from build123d import *

# Parameters (mm, degrees)
F1_DEPTH    = 6
F2_F1_R     = 0.2
F2_F2_R     = 0.2
F3_T4_DEPTH = 28.4585903453
F3_T9_DEPTH = 28.4585903453
F4_R        = 5.99999


# Not quite as in the source:
# - a fillet or chamfer that OpenCascade refuses, or shapes differently, is made with other operations: its cross-section is extruded or revolved along the edge and cut away or added
# - a fillet or chamfer is up to 0.001 mm smaller than in the source, because OpenCascade refuses the exact size


with BuildPart() as f1:
    # F0 (on Top) → F1 (new body)
    with BuildSketch(Plane.XY):
        Polygon((-7.5, 8), (-4.418584287, -3.5), (4.418584287, -3.5), (7.5, 8), align=None)
        with BuildLine():
            ThreePointArc((-1.5, 1.5), (-2.5606601718, 4.0606601718), (0, 3))
            ThreePointArc((0, 3), (2.5606601718, 4.0606601718), (1.5, 1.5))
            ThreePointArc((1.5, 1.5), (2.5606601718, -1.0606601718), (0, 0))
            ThreePointArc((0, 0), (-2.5606601718, -1.0606601718), (-1.5, 1.5))
        make_face(mode=Mode.SUBTRACT)
        Polygon((-9, -5), (-9, -7), (9, -7), (9, -5), (4.0166604984, -5), (-4.0166604984, -5), align=None)
        Polygon((-4.418584287, -3.5), (-4.0166604984, -5), (4.0166604984, -5), (4.418584287, -3.5), align=None)
    extrude(amount=F1_DEPTH)

    # F2: fillet of radius 0.2 on 4 edges, made by hand

    # F2_f1
    f2_f1_edges = [f1.edges().sort_by_distance(p)[0] for p in [
        (-1.5, 1.5, 3),
        (0, 3, 3),
        (1.5, 1.5, 3),
    ]]
    fillet(f2_f1_edges, radius=F2_F1_R)

    # F2_f2
    f2_f2_edges = [f1.edges().sort_by_distance(p)[0] for p in [
        (0, 0, 3),
    ]]
    fillet(f2_f2_edges, radius=F2_F2_R)

    # F3: fillet of radius 3 on 2 edges, made by hand


with BuildPart() as f3_tool2:
    # F3_s3 → F3_t4 (new body)
    with BuildSketch(Plane(origin=(-4.4435475741, 16.5835453123, 0), x_dir=(0, 0, 1), z_dir=(0.2588190451, -0.9659258263, 0))):
        with BuildLine():
            ThreePointArc((3, 5.1738913363), (5.1213203436, 4.2952116799), (6, 2.1738913363))
            Line((6, 2.1738913363), (6, 5.1738913363))
            Line((6, 5.1738913363), (3, 5.1738913363))
        make_face()
    extrude(amount=F3_T4_DEPTH)

    split(bisect_by=Plane.XZ.offset(5), keep=Keep.BOTTOM)


with BuildPart() as f1_1:
    add(f1.part)

    # F3_t1: cut F3_tool2
    add(f3_tool2.part, mode=Mode.SUBTRACT)


with BuildPart() as f3_tool7:
    # F3_s8 → F3_t9 (new body)
    with BuildSketch(Plane(origin=(-2.9220776041, -10.905342082, 0), x_dir=(0, 0, 1), z_dir=(0.2588190451, 0.9659258263, 0))):
        with BuildLine():
            ThreePointArc((3, 5.1738913363), (5.1213203436, 4.2952116799), (6, 2.1738913363))
            Line((6, 2.1738913363), (6, 5.1738913363))
            Line((6, 5.1738913363), (3, 5.1738913363))
        make_face()
    extrude(amount=F3_T9_DEPTH)

    split(bisect_by=Plane.XZ.offset(5), keep=Keep.BOTTOM)


with BuildPart() as f1_2:
    add(f1_1.part)

    # F3_t6: cut F3_tool7
    add(f3_tool7.part, mode=Mode.SUBTRACT)

    # F4 (radius 6 in the source; OpenCascade refuses exactly that, so slightly less here)
    f4_edges = [f1_2.edges().sort_by_distance(p)[0] for p in [
        (9, -6, 6),
        (-9, -6, 6),
    ]]
    fillet(f4_edges, radius=F4_R)

    # F5: F1 across plane


with BuildPart() as f1_3:
    add(f1_2.part)
    add(f1_2.part.mirror(Plane.XY))


solid = f1_3.part
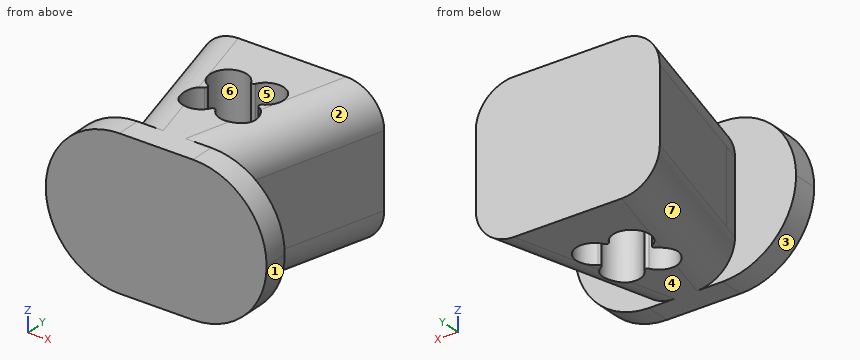
The listing builds one solid part. Answer for the finished solid, in the listing's coordinates (mm). Face numbers are marked on the shaded views. A direction names the side the tool comes from. Give positions to 0.01 mm unless a question says otherwise; leave off trailing zeros.
Item 1: A tool of negligible diameter and unlimited length cuts with its end or side. For the marked faces 1, 2 and 3, from which of +Z, -Z, +X, -X, +Y, -Y can it reach the whole face along a straight path? Write none if from no direction.
Derived:
face 1: -Z, +X, -Y
face 2: +Z, +X
face 3: -Z, -X, -Y
Item 2: Determine the mould class of the marked faces 4, 5, 6 and 7 for opening direction X: +X half, -X half, draft (parallel to the pull), parting line (faces both ways), or undercut.
Derived:
face 4: draft
face 5: undercut
face 6: undercut
face 7: -X half
Item 3: Each of these flat-tipped pins is pushed along its axis until it touches: pin 1 Ø4 at (y, z) = (3, 1.5) entering from +X; pin 2 Ø3 at (x, y) = (-3, -4) entering from +Z; pin 3 Ø4 at (y, z) = (5, 0) entering from -X. Where does it stop, or does it pass through?
Derived:
pin 1: stops at x = 6.7
pin 2: stops at z = 6
pin 3: stops at x = -7.23
Item 4: Find the intervals of material crossed by line 1 along Y through (x, z) = (1.5, 1.25); line 2 along X through (y, z) = (4.25, -3); line 3 along Y through (x, z) = (-2.25, -2.5), in increasing order.
Derived:
line 1: y = -7 to -1.5, 4.5 to 8
line 2: x = -6.5 to -2.33, -0.67 to 0.67, 2.33 to 6.5
line 3: y = -7 to -1.3, 1.3 to 1.7, 4.3 to 8
